Design review of the part built by this model. Coordinates are the model's own, in mm. Face numbers are marked on the shaded views. A direction names the side the tool comes from. Coordinates: 2 decimals unless noted, no trailing zeros. Loops run counter-clockwise (first coordinate to the right, second up) from the corner with the lowest first, then second, coordinate; pieces in that order, holes last. Notation, with made-up numbers: (-39.5, 31) - (-2.5, 31) arc R9 cw to (-2.5, 42) - close; hole circle Ø2 at (72.5, -17.5). An arc over 180 degrees is marked (long way). Use one line per item in the form item = value. Start each with the question number.
(1) Add section A-A (y = -7). State the section outline as (x, z) points, plus the area to 3 significant figures.
(2) Tool access review of the marked faces 1, 2 and 3: name each direction out of +Z, -Z, +X, -X, +Y, -Y from which nothing blocks a thin tool from reaching the whole face with its end or side.
(3) Clearance check with flat-ended pins moving along their axes: pin 1 Ø2.5 at (x, z) = (-6.5, 24) entering from +Y; pin 2 Ø1.1 at (x, z) = (-4.5, 20) entering from -Y; pin 3 Ø5 at (x, z) = (0, 31.6) entering from -Y. State where each tip first meets the part, or that it passes through.
(4) Add section D-D (z = 7). State the section outline as (x, y) points, plus the area to 3 significant figures.
(5) Add section C-C (y = -12.25). State the section outline as (x, z) points, plus the area to 3 significant figures.
(6) The part is to be moulded in two halves that separate along X. For the marked faces 4, 5 and 6, say which applies: pulls with the +X half, pulls with the -X half, needs draft (parallel to the pull), parting line crosses it, or undercut.
(7) Add section B-B (x = 0). State the section outline as (y, z) points.
(8) For L1, parallel to Z at x = 0, y = -6.75; L2, parallel to Y at x = -2.5, z = 14.5; L3, parallel to Z at x = 0, y = -16.65, list the stretches that pass through material, from the lowest coordinate up.
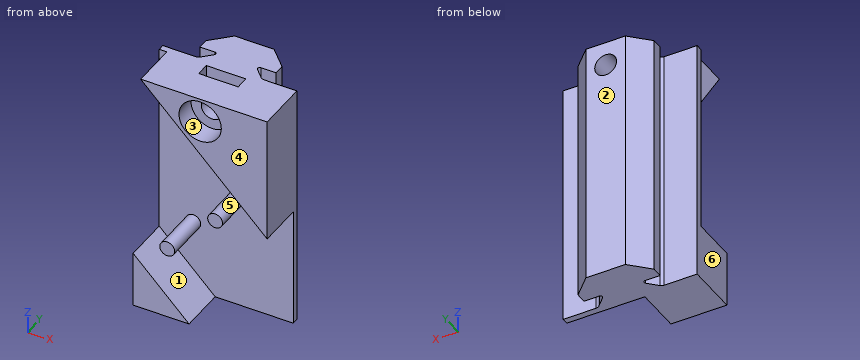
Autodesk Fusion 360 part; units mm, degrees
sketch "Sketch1" plane through (0, 0, 0) normal (0, 0, 1) x (1, 0, 0)
  line L0 (10, 4.8314) -> (10, 9.5)
  line L1 (-4.4022, -9.8222) -> (-3.1214, -8.5414)
  arc A0 (3.2628, -8.2) -> (3.1214, -8.5414) centre (3.2628, -8.4) ccw
  line L2 (-5.5, 6.5607) -> (-5.5, 8.2)
  line L3 (-5.5, -6.5607) -> (-2.8393, -3.9)
  line L4 (-4.8314, 10) -> (-9.5, 10)
  line L5 (2.8393, 3.9) -> (-2.8393, 3.9)
  arc A1 (-10, -9.5) -> (-9.5, -10) centre (-9.5, -9.5) ccw
  line L6 (9.5, 10) -> (4.8314, 10)
  arc A2 (-3.2628, 8.2) -> (-3.1214, 8.5414) centre (-3.2628, 8.4) ccw
  line L7 (-8.2, 3.2628) -> (-8.2, 5.5)
  line L8 (2.8393, -3.9) -> (5.5, -6.5607)
  line L9 (-10, 9.5) -> (-10, 4.9)
  arc A3 (9.5, -10) -> (10, -9.5) centre (9.5, -9.5) ccw
  line L10 (-6.5607, -5.5) -> (-8.2, -5.5)
  line L11 (3.1214, -8.5414) -> (4.2336, -9.6536)
  line L12 (-8.2, -5.5) -> (-8.2, -3.2628)
  line L13 (-9.9987, -4.7917) -> (-10, -9.5)
  line L14 (10, -9.5) -> (10, -4.8314)
  line L15 (3.2628, 8.2) -> (5.5, 8.2)
  arc A4 (8.5414, -3.1214) -> (8.2, -3.2628) centre (8.4, -3.2628) ccw
  arc A5 (-3.1214, -8.5414) -> (-3.2628, -8.2) centre (-3.2628, -8.4) ccw
  line L16 (4.8314, -10) -> (9.5, -10)
  line L17 (-3.9, -2.8393) -> (-6.5607, -5.5)
  line L18 (-3.2628, -8.2) -> (-5.5, -8.2)
  line L19 (3.9, 2.8393) -> (6.5607, 5.5)
  line L20 (-3.1214, 8.5414) -> (-4.4312, 9.8494)
  line L21 (8.2, -5.5) -> (6.5607, -5.5)
  arc A6 (-10, 4.9) -> (-9.8494, 4.4312) centre (-9.3734, 4.8428) ccw
  line L22 (8.5414, 3.1214) -> (9.8222, 4.4022)
  circle A7 centre (0, 0) radius 2.1
  line L23 (3.9, -2.8393) -> (3.9, 2.8393)
  line L24 (6.5607, -5.5) -> (3.9, -2.8393)
  line L25 (5.5, -6.5607) -> (5.5, -8.2)
  line L26 (8.2, -3.2628) -> (8.2, -5.5)
  arc A8 (10, -4.8314) -> (9.8222, -4.4022) centre (9.3929, -4.8314) ccw
  line L27 (-5.5, -8.2) -> (-5.5, -6.5607)
  arc A9 (-4.8314, -10) -> (-4.4022, -9.8222) centre (-4.8314, -9.3929) ccw
  line L28 (5.5, -8.2) -> (3.2628, -8.2)
  line L29 (9.8222, -4.4022) -> (8.5414, -3.1214)
  arc A10 (-9.8222, -4.4022) -> (-9.9987, -4.7917) centre (-9.3929, -4.8314) ccw
  line L30 (-8.5414, -3.1214) -> (-9.8222, -4.4022)
  arc A11 (4.2336, -9.6536) -> (4.8314, -10) centre (4.8837, -9.2207) ccw
  arc A12 (-8.2, -3.2628) -> (-8.5414, -3.1214) centre (-8.4, -3.2628) ccw
  line L31 (-9.5, -10) -> (-4.8314, -10)
  line L32 (-2.8393, -3.9) -> (2.8393, -3.9)
  line L33 (-5.8557, 10) -> (6.4454, 10) construction
  arc A13 (10, 9.5) -> (9.5, 10) centre (9.5, 9.5) ccw
  arc A14 (3.1214, 8.5414) -> (3.2628, 8.2) centre (3.2628, 8.4) ccw
  line L34 (-5.5, 8.2) -> (-3.2628, 8.2)
  line L35 (-3.9, 2.8393) -> (-3.9, -2.8393)
  line L36 (4.4022, 9.8222) -> (3.1214, 8.5414)
  arc A15 (4.8314, 10) -> (4.4022, 9.8222) centre (4.8314, 9.3929) ccw
  line L37 (-9.8494, 4.4312) -> (-8.5414, 3.1214)
  line L38 (5.5, 8.2) -> (5.5, 6.5607)
  line L39 (6.5607, 5.5) -> (8.2, 5.5)
  arc A16 (-8.5414, 3.1214) -> (-8.2, 3.2628) centre (-8.4, 3.2628) ccw
  line L40 (8.2, 5.5) -> (8.2, 3.2628)
  arc A17 (-4.4312, 9.8494) -> (-4.8314, 10) centre (-4.8314, 9.3929) ccw
  line L41 (-8.2, 5.5) -> (-6.5607, 5.5)
  arc A18 (9.8222, 4.4022) -> (10, 4.8314) centre (9.3929, 4.8314) ccw
  arc A19 (-9.5, 10) -> (-10, 9.5) centre (-9.5, 9.5) ccw
  line L42 (-2.8393, 3.9) -> (-5.5, 6.5607)
  line L43 (-6.5607, 5.5) -> (-3.9, 2.8393)
  arc A20 (8.2, 3.2628) -> (8.5414, 3.1214) centre (8.4, 3.2628) ccw
  line L44 (5.5, 6.5607) -> (2.8393, 3.9)
  line L45 (5.4, -6.6021) -> (5.4, -8.1)
  line L46 (5.4, -8.1) -> (3.2628, -8.1)
  arc A21 (3.2628, -8.1) -> (3.0507, -8.6121) centre (3.2628, -8.4) ccw
  line L47 (3.0507, -8.6121) -> (4.1561, -9.7175)
  arc A22 (4.1561, -9.7175) -> (4.8282, -10.1) centre (4.8837, -9.2207) ccw
  line L48 (4.8282, -10.1) -> (9.5, -10.1)
  arc A23 (9.5, -10.1) -> (10.1, -9.5) centre (9.5, -9.5) ccw
  line L49 (10.1, -9.5) -> (10.1, -4.8314)
  arc A24 (10.1, -4.8314) -> (9.8929, -4.3315) centre (9.3929, -4.8314) ccw
  line L50 (9.8929, -4.3315) -> (8.6121, -3.0507)
  arc A25 (8.6121, -3.0507) -> (8.1, -3.2628) centre (8.4, -3.2628) ccw
  line L51 (8.1, -3.2628) -> (8.1, -5.4)
  line L52 (8.1, -5.4) -> (6.6021, -5.4)
  line L53 (6.6021, -5.4) -> (4, -2.7979)
  line L54 (4, -2.7979) -> (4, 2.7979)
  line L55 (4, 2.7979) -> (6.6021, 5.4)
  line L56 (6.6021, 5.4) -> (8.1, 5.4)
  line L57 (8.1, 5.4) -> (8.1, 3.2628)
  arc A26 (8.1, 3.2628) -> (8.6121, 3.0507) centre (8.4, 3.2628) ccw
  line L58 (8.6121, 3.0507) -> (9.8929, 4.3315)
  arc A27 (9.8929, 4.3315) -> (10.1, 4.8314) centre (9.3929, 4.8314) ccw
  line L59 (10.1, 4.8314) -> (10.1, 9.5)
  arc A28 (10.1, 9.5) -> (9.5, 10.1) centre (9.5, 9.5) ccw
  line L60 (9.5, 10.1) -> (4.8314, 10.1)
  arc A29 (4.8314, 10.1) -> (4.3315, 9.8929) centre (4.8314, 9.3929) ccw
  line L61 (4.3315, 9.8929) -> (3.0507, 8.6121)
  arc A30 (3.0507, 8.6121) -> (3.2628, 8.1) centre (3.2628, 8.4) ccw
  line L62 (3.2628, 8.1) -> (5.4, 8.1)
  line L63 (5.4, 8.1) -> (5.4, 6.6021)
  line L64 (5.4, 6.6021) -> (2.7979, 4)
  line L65 (2.7979, 4) -> (-2.7979, 4)
  line L66 (-2.7979, 4) -> (-5.4, 6.6021)
  line L67 (-5.4, 6.6021) -> (-5.4, 8.1)
  line L68 (-5.4, 8.1) -> (-3.2628, 8.1)
  arc A31 (-3.2628, 8.1) -> (-3.0509, 8.6124) centre (-3.2628, 8.4) ccw
  line L69 (-3.0509, 8.6124) -> (-4.3627, 9.9223)
  arc A32 (-4.3627, 9.9223) -> (-4.8314, 10.1) centre (-4.8314, 9.3929) ccw
  line L70 (-4.8314, 10.1) -> (-9.5, 10.1)
  arc A33 (-9.5, 10.1) -> (-10.1, 9.5) centre (-9.5, 9.5) ccw
  line L71 (-10.1, 9.5) -> (-10.1, 4.9044)
  arc A34 (-10.1, 4.9044) -> (-9.9226, 4.363) centre (-9.3734, 4.8428) ccw
  line L72 (-9.9226, 4.363) -> (-8.6124, 3.0509)
  arc A35 (-8.6124, 3.0509) -> (-8.1, 3.2628) centre (-8.4, 3.2628) ccw
  line L73 (-8.1, 3.2628) -> (-8.1, 5.4)
  line L74 (-8.1, 5.4) -> (-6.6021, 5.4)
  line L75 (-6.6021, 5.4) -> (-4, 2.7979)
  line L76 (-4, 2.7979) -> (-4, -2.7979)
  line L77 (-4, -2.7979) -> (-6.6021, -5.4)
  line L78 (-6.6021, -5.4) -> (-8.1, -5.4)
  line L79 (-8.1, -5.4) -> (-8.1, -3.2628)
  arc A36 (-8.1, -3.2628) -> (-8.6121, -3.0507) centre (-8.4, -3.2628) ccw
  line L80 (-8.6121, -3.0507) -> (-9.8929, -4.3315)
  arc A37 (-9.8929, -4.3315) -> (-10.0987, -4.7886) centre (-9.3929, -4.8314) ccw
  line L81 (-10.0987, -4.7886) -> (-10.1, -9.4997)
  arc A38 (-10.1, -9.4997) -> (-9.5, -10.1) centre (-9.5, -9.5) ccw
  line L82 (-9.5, -10.1) -> (-4.8314, -10.1)
  arc A39 (-4.8314, -10.1) -> (-4.3315, -9.8929) centre (-4.8314, -9.3929) ccw
  line L83 (-4.3315, -9.8929) -> (-3.0507, -8.6121)
  arc A40 (-3.0507, -8.6121) -> (-3.2628, -8.1) centre (-3.2628, -8.4) ccw
  line L84 (-3.2628, -8.1) -> (-5.4, -8.1)
  line L85 (-5.4, -8.1) -> (-5.4, -6.6021)
  line L86 (-5.4, -6.6021) -> (-2.7979, -4)
  line L87 (-2.7979, -4) -> (2.7979, -4)
  line L88 (2.7979, -4) -> (5.4, -6.6021)
  line L89 (-9.5, -9.5) -> (9.5, -9.5)
  line L90 (9.5, -9.5) -> (9.5, -17.5)
  line L91 (9.5, -17.5) -> (-9.5, -17.5)
  line L92 (-9.5, -17.5) -> (-9.5, -9.5)
  dimension "d1" = 0.1
  dimension "d2" = 8
extrude "Extrude1" add sketch "Sketch1" along normal blind 35 contours L47 A22 L48 L82 A39 L83 L89 L90 L91 L92 | L45 L46 A21 L47 L83 A40 L84 L85 L86 L87 L88 L89
sketch "Sketch2" plane through (0, -17.5, 0) normal (0, -1, 0) x (1, 0, 0)
  line L0 (-9.5, 0) -> (9.5, 0)
  line L1 (9.5, 0) -> (9.5, 35)
  line L2 (9.5, 35) -> (-9.5, 35)
  line L3 (-9.5, 35) -> (-9.5, 0)
  line L4 (13.7568, 12.4504) -> (-13.7568, 12.5496) construction
  line L5 (0.3182, 26.2532) -> (13.7532, 12.8182)
  line L6 (13.7532, 12.8182) -> (-0.3182, -1.2532)
  line L7 (-0.3182, -1.2532) -> (-13.7532, 12.1818)
  line L8 (-13.7532, 12.1818) -> (0.3182, 26.2532)
  line L9 (0.3182, 26.2532) -> (-0.3182, -1.2532) construction
  line L10 (13.7532, 12.8182) -> (-13.7532, 12.1818) construction
  line L11 (-13.7532, 12.1818) -> (-8.3085, 6.7371) construction
  line L12 (-8.3085, 6.7371) -> (5.7629, 20.8085) construction
  line L13 (-8.3085, 6.7371) -> (-4.6669, 10.3787) construction
  line L14 (-4.6669, 10.3787) -> (2.1213, 17.1669) construction
  line L15 (2.1213, 17.1669) -> (5.7629, 20.8085) construction
  line L16 (2.1213, 17.1669) -> (5.7629, 20.8085) construction
  circle A0 centre (2.1213, 17.1669) radius 1.05
  circle A1 centre (-4.6669, 10.3787) radius 1.05
  line L17 (0.3182, 26.2532) -> (-8.4286, 35)
  point P0 (0, 12.5)
  dimension "d15" = 19.9
  dimension "d16" = 7.7
  dimension "d17" = 5.15
  dimension "d18" = 9.6
  dimension "d19" = 5.15
  dimension "d20" = 2.1
  dimension "d21" = 2.1
extrude "Extrude2" cut sketch "Sketch2" against normal blind 6.5 contours L0 L1 L3 L5 L6 L7 L8 | L0 L1 L6 | L2 L3 L8 L17
sketch "Sketch3" plane through (0, -17.5, 0) normal (0, -1, 0) x (1, 0, 0)
  line L0 (-8.4286, 35) -> (9.5, 17.0714)
  line L1 (9.5, 17.0714) -> (9.5, 35)
  line L2 (9.5, 35) -> (-8.4286, 35)
  line L3 (9.5, 35) -> (0, 35) construction
  circle A0 centre (0, 31.6) radius 1.55
  circle A1 centre (0, 31.6) radius 3
  dimension "d22" = 3.1
  dimension "d23" = 6
extrude "Extrude3" cut sketch "Sketch3" against normal blind 20 contours A0
extrude "Extrude4" cut sketch "Sketch3" against normal blind 3 contours A1
sketch "Sketch4" plane through (0, 0, 35) normal (0, 0, 1) x (-1, 0, 0)
  line L0 (8.4286, 11) -> (8.4286, 17.5)
  line L1 (8.4286, 17.5) -> (-9.5, 17.5)
  line L2 (-9.5, 17.5) -> (-9.5, 10.1)
  line L3 (-9.5, 10.1) -> (-4.8282, 10.1)
  arc A0 (-4.1561, 9.7175) -> (-4.8282, 10.1) centre (-4.8837, 9.2207) ccw
  line L4 (-4.1561, 9.7175) -> (-3.0507, 8.6121)
  arc A1 (-3.2628, 8.1) -> (-3.0507, 8.6121) centre (-3.2628, 8.4) ccw
  line L5 (-3.2628, 8.1) -> (-5.4, 8.1)
  line L6 (-5.4, 8.1) -> (-5.4, 6.6021)
  line L7 (-5.4, 6.6021) -> (-2.7979, 4)
  line L8 (-2.7979, 4) -> (2.7979, 4)
  line L9 (2.7979, 4) -> (5.4, 6.6021)
  line L10 (5.4, 6.6021) -> (5.4, 8.1)
  line L11 (5.4, 8.1) -> (3.2628, 8.1)
  arc A2 (3.0507, 8.6121) -> (3.2628, 8.1) centre (3.2628, 8.4) ccw
  line L12 (3.0507, 8.6121) -> (4.3315, 9.8929)
  arc A3 (4.8314, 10.1) -> (4.3315, 9.8929) centre (4.8314, 9.3929) ccw
  line L13 (4.8314, 10.1) -> (9.5, 10.1)
  line L14 (9.5, 10.1) -> (9.5, 11)
  line L15 (9.5, 11) -> (8.4286, 11)
  line L16 (0, 4) -> (0, 17.5) construction
  line L17 (2.8, 12.95) -> (-2.8, 12.95)
  line L18 (-2.8, 12.95) -> (-2.8, 11.05)
  line L19 (-2.8, 11.05) -> (2.8, 11.05)
  line L20 (2.8, 11.05) -> (2.8, 12.95)
  line L21 (2.8, 12.95) -> (-2.8, 11.05) construction
  line L22 (-2.8, 12.95) -> (2.8, 11.05) construction
  point P0 (0, 12)
  point P1 (0, 17.5)
  dimension "d28" = 5.6
  dimension "d29" = 1.9
  dimension "d30" = 5.5
extrude "Extrude5" cut sketch "Sketch4" against normal blind 6.5 contours L17 L18 L19 L20
Computed values:
q1.outline = (-5.4, 0) - (5.4, 0) - (5.4, 35) - (-5.4, 35) - close; hole circle Ø3.1 at (0, 31.6)
q1.area = 370 mm^2
q2.face_1 = +X, -Y
q2.face_2 = +Z, -Z, +X, -X, +Y
q2.face_3 = -Y
q3.pin_1 = -6.45
q3.pin_2 = -11
q3.pin_3 = -14.5
q4.outline = (-9.5, -17.5) - (-8.57, -17.5) - (-8.57, -11) - (9.5, -11) - (9.5, -10.1) - (4.83, -10.1) arc R0.88 cw to (4.16, -9.72) - (3.05, -8.61) arc R0.3 cw to (3.26, -8.1) - (5.4, -8.1) - (5.4, -6.6) - (2.8, -4) - (-2.8, -4) - (-5.4, -6.6) - (-5.4, -8.1) - (-3.26, -8.1) arc R0.3 cw to (-3.05, -8.61) - (-4.33, -9.89) arc R0.71 cw to (-4.83, -10.1) - (-9.5, -10.1) - close
q4.area = 75.0 mm^2
q5.outline = (-9.5, 0) - (-1.57, 0) - (-9.5, 7.93) - close; (-8.43, 35) - (-2.8, 29.37) - (-2.8, 35) - close; circle Ø2.1 at (-4.67, 10.38); (-1.93, 28.5) - (9.5, 17.07) - (9.5, 35) - (2.8, 35) - (2.8, 28.5) - close; circle Ø2.1 at (2.12, 17.17)
q5.area = 163 mm^2
q6.face_4 = needs draft
q6.face_5 = undercut
q6.face_6 = pulls with the -X half
q7.outline = (-17.5, 26.57) - (-11, 26.57) - (-11, 0) - (-4, 0) - (-4, 30.05) - (-11.05, 30.05) - (-11.05, 28.5) - (-12.95, 28.5) - (-12.95, 30.05) - (-14.5, 30.05) - (-14.5, 28.6) - (-17.5, 28.6) - close; (-17.5, 34.6) - (-14.5, 34.6) - (-14.5, 33.15) - (-12.95, 33.15) - (-12.95, 35) - (-17.5, 35) - close; (-11.05, 33.15) - (-4, 33.15) - (-4, 35) - (-11.05, 35) - close
q8.L1 = 0 to 30.05, 33.15 to 35
q8.L2 = -11 to -4
q8.L3 = 26.57 to 28.6, 34.6 to 35
